```python
from build123d import *

# Parameters (mm, degrees)
SKETCH_1_W      = 55
SKETCH_1_H      = 55
EXTRUDE_1_DEPTH = 66
SKETCH_2_W      = 10
SKETCH_2_H      = 7
EXTRUDE_2_DEPTH = 5


with BuildPart() as part:
    # 草图1 → 凸台-拉伸1 (new body)
    with BuildSketch(Plane(origin=(0, 0, 0), x_dir=(1, 0, 0), z_dir=(0, 1, 0))):
        Rectangle(SKETCH_1_W, SKETCH_1_H)
    extrude(amount=EXTRUDE_1_DEPTH)

    # 草图2 → 凸台-拉伸2 (add)
    with BuildSketch(Plane.XY.offset(27.5)):
        with Locations((0, 62.5)):
            Rectangle(SKETCH_2_W, SKETCH_2_H)
    extrude(amount=EXTRUDE_2_DEPTH)


solid = part.part
```
Design review of the part built by this model. Coordinates are the model's own, in mm. A direction names the side the tool comes from. Round coordinates to 2 decimals unless told otherwise and drop trailing zeros. Write each loop counter-clockwise with the first axis right and the second up, starting at its lowest first coordinate (ties: lowest second). Pieces come first, ordered by that corner, then holes.
Item 1: For probe 1 along Z at (x, y) = (-2.5, 51.5), list the stretches that pass through material, from the lowest coordinate up.
Item 2: Clearance check with flat-ended pins moving along their axes: pin 1 Ø2.5 at (y, z) = (61, 29.5) entering from -X; pin 2 Ø2 at (x, y) = (-2, 49) entering from +Z; pin 3 Ø2.5 at (x, z) = (2.5, 29.5) entering from -Y. State where each tip first meets the part, or that it passes through.
Item 3: We need section C-C on y = 10.5. Write out the cut boundary in (x, z), and give its area (4 significant figures).
Item 4: For faces 1 (the flat face through (0, 33, -27.5)), 2 (the flat face through (0, 59, 30)), 3 (the flat face through (5, 62, 30)), 4 (the flat face through (-5, 62, 30)), list the 3-axis set-ups (+Z, -Z, +X, -X, +Y, -Y) from which the entire face can be reached by the end or side of a thin tool; tool diameter is ignored.
Item 5: We need section B-B on z = 28.5. Write out the cut boundary in (x, y).
Item 6: We need section A-A on x = 1. Write out the cut boundary in (y, z), and give its area (4 significant figures).
Returned:
1. probe 1: z = -27.5 to 27.5
2. pin 1: stops at x = -5
2. pin 2: stops at z = 27.5
2. pin 3: stops at y = 59
3. outline: (-27.5, -27.5) - (27.5, -27.5) - (27.5, 27.5) - (-27.5, 27.5) - close
3. area: 3,025 mm2
4. face 1: -Z, +X, -X, +Y, -Y
4. face 2: +Z, +X, -X, -Y
4. face 3: +Z, +X, +Y, -Y
4. face 4: +Z, -X, +Y, -Y
5. outline: (-5, 59) - (5, 59) - (5, 66) - (-5, 66) - close
6. outline: (0, -27.5) - (66, -27.5) - (66, 32.5) - (59, 32.5) - (59, 27.5) - (0, 27.5) - close
6. area: 3,665 mm2
